Could you check a few things on this model? Use its own coordinates, in mm. Give positions to 0.01 mm unless a question says otherwise; leave off trailing zeros. Write each loop counter-clockwise with the first axis right and the second up, starting at its lowest first coordinate (ties: lowest second). Pieces come first, ordered by that corner, then holes. Notation, with made-up numbers: M -17,37.5 L 19,37.5 A15 ccw 19,56.5 Z; hole C 75,8 d2. An arc over 180 degrees is marked long. Use one line per item in the form item = value.
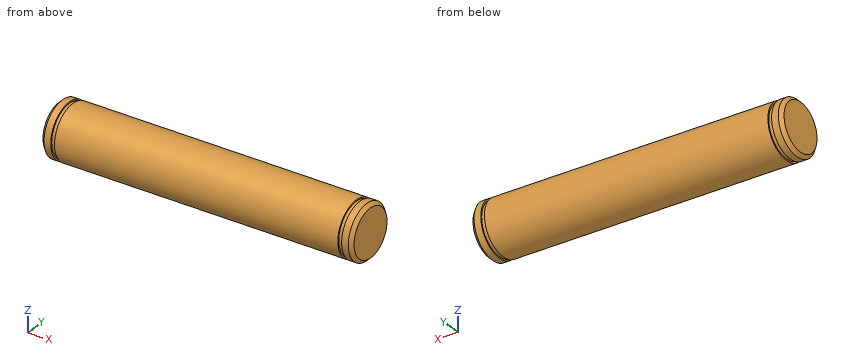
from build123d import *

# Parameters (mm, degrees)
F2_SIZE = 1


with BuildPart() as f1:
    # F0 (on Front) → F1 (revolve)
    with BuildSketch(Plane.XZ):
        Polygon((42, 8), (0, 8), (-42, 8), (-42, 7.6), (-43.1, 7.6), (-43.1, 8), (-46.1, 8), (-46.1, 0), (46.1, 0), (46.1, 8), (43.1, 8), (43.1, 7.6), (42, 7.6), align=None)
    revolve(axis=Axis((0, 0, 0), (1, 0, 0)))

    # F2
    f2_edges = [f1.edges().sort_by_distance(p)[0] for p in [
        (-46.1, 0, -8),
        (46.1, 0, -8),
    ]]
    chamfer(f2_edges, length=F2_SIZE)


solid = f1.part
1) I want a section at A-A, the plane x = 36. Please give me the cut outline in (y, z).
Checked values:
outline = C 0,0 d16
2) If I drill on L1, parallel to X at y = 6.5, z = -4; L2, parallel to Y at x = 9, z = -0.25; L3, parallel to Z at x = 22.5, y = -0.5, over which ranges is the centre line in solid material (lowest first)?
Checked values:
L1 = -45.47 to -43.1, -42 to 42, 43.1 to 45.47
L2 = -8 to 8
L3 = -7.98 to 7.98
3) For pin 1 Ø5 at (x, y) = (-3, -0.5) entering from +Z; pin 2 Ø2 at (x, z) = (13.5, 4) entering from -Y; pin 3 Ø1 at (x, y) = (-18.5, -6) entering from -Z, each with a flat end and sliding along its axis, tell me the tip position at first contact or that it passes through.
Checked values:
pin_1 = 8
pin_2 = -7.42
pin_3 = -5.81
